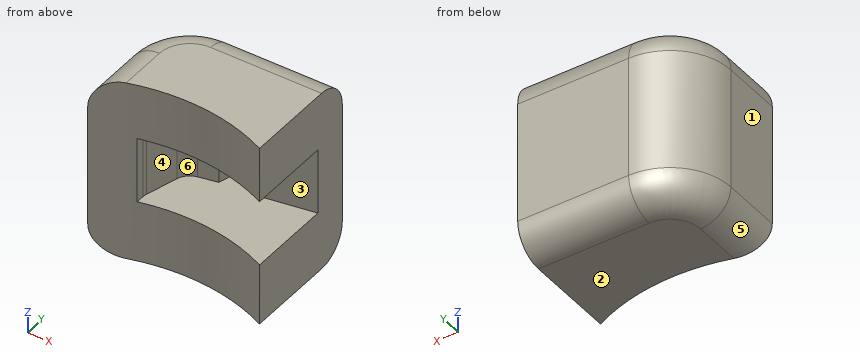
```python
from build123d import *

# Parameters (mm, degrees)
SKETCH1_W                      = 60
SKETCH1_H                      = 60
BOSS_EXTRUDE1_DEPTH            = 40
SKETCH2_R                      = 65
CUT_EXTRUDE1_DEPTH             = 82.241203775
CAVITY1_START                  = -9.816541319
CAVITY1_DEPTH                  = 21.6
SKETCH3_W                      = 21.6
SKETCH3_H                      = 10.847854466
CUT_EXTRUDE2_DEPTH             = 10
SKETCH4_W                      = 60
SKETCH4_H                      = 40
CUT_EXTRUDE3_DEPTH             = 2.5
SKETCH5_W                      = 60
SKETCH5_H                      = 40
CUT_EXTRUDE4_DEPTH             = 1
FILLET1_R                      = 20
FILLET2_R                      = 10
SKETCH6_W                      = 16.032155739
SKETCH6_H                      = 21.6
CUT_EXTRUDE5_DEPTH             = 58.845323025
CUT_EXTRUDE5_DIRECTION_2_REACH = 59.845


# Read off the part's stored shape, not the designer's step: Cavity1
with BuildPart() as part:
    # Sketch1 → Boss-Extrude1 (new body)
    with BuildSketch(Plane(origin=(0, 0, 0), x_dir=(1, 0, 0), z_dir=(0, 1, 0))):
        with Locations((7.418353663, 0)):
            Rectangle(SKETCH1_W, SKETCH1_H)
    extrude(amount=BOSS_EXTRUDE1_DEPTH)

    # Sketch2 → Cut-Extrude1 (cut, through all)
    with BuildSketch(Plane.XY.offset(30)):
        with Locations((8.211917099, -58.463187122)):
            Circle(SKETCH2_R)
    extrude(amount=-CUT_EXTRUDE1_DEPTH, mode=Mode.SUBTRACT)

    # Cavity1 outline → Cavity1 (cut)
    with BuildSketch(Plane.XY.offset(CAVITY1_START)):
        with BuildLine():
            Line((37.418353663, 28.401179965), (19.900272044, 25.583077508))
            Line((19.900272044, 25.583077508), (10.402665556, 28.20897422))
            Line((10.402665556, 28.20897422), (11.046955399, 30.539306317))
            Line((11.046955399, 30.539306317), (8.306376045, 31.297021255))
            Line((8.306376045, 31.297021255), (6.40567059, 24.42235921))
            Line((6.40567059, 24.42235921), (0.254542205, 23.221419402))
            ThreePointArc((0.254542205, 23.221419402), (-2.379423034, 21.883873023), (-3.91543957, 19.360491087))
            Line((-3.91543957, 19.360491087), (-6.809482783, 8.89302545))
            ThreePointArc((-6.809482783, 8.89302545), (-6.970209101, 6.844246899), (-6.353840253, 4.883783703))
            ThreePointArc((-6.353840253, 4.883783703), (14.742582186, 6.207906989), (35.148358053, 0.692777486))
            Line((35.148358053, 0.692777486), (37.418353663, 2.423285883))
            Line((37.418353663, 2.423285883), (37.418353663, 28.401179965))
        make_face()
    extrude(amount=CAVITY1_DEPTH, mode=Mode.SUBTRACT)

    # Sketch3 → Cut-Extrude2 (cut)
    with BuildSketch(Plane(origin=(37.418353663, 0, 0), x_dir=(0, 0, -1), z_dir=(1, 0, 0))):
        with Locations((-0.983458681, 5.423927233)):
            Rectangle(SKETCH3_W, SKETCH3_H)
    extrude(amount=-CUT_EXTRUDE2_DEPTH, mode=Mode.SUBTRACT)

    # Sketch4 → Cut-Extrude3 (cut)
    with BuildSketch(Plane.ZY.offset(22.581646337)):
        with Locations((0, 20)):
            Rectangle(SKETCH4_W, SKETCH4_H)
    extrude(amount=-CUT_EXTRUDE3_DEPTH, mode=Mode.SUBTRACT)

    # Sketch5 → Cut-Extrude4 (cut)
    with BuildSketch(Plane(origin=(37.418353663, 0, 0), x_dir=(0, 0, -1), z_dir=(1, 0, 0))):
        with Locations((0, 20)):
            Rectangle(SKETCH5_W, SKETCH5_H)
    extrude(amount=-CUT_EXTRUDE4_DEPTH, mode=Mode.SUBTRACT)

    # Fillet1
    fillet1_edges = [part.edges().sort_by_distance(p)[0] for p in [
        (-20.081646337, 40, 0),
    ]]
    fillet(fillet1_edges, radius=FILLET1_R)

    # Fillet2
    fillet2_edges = [part.edges().sort_by_distance(p)[0] for p in [
        (-20.081646337, 10.027910314, 30),
        (18.168353663, 40, -30),
        (-20.081646337, 10.027910314, -30),
        (-14.22378196, 34.142135624, -30),
        (18.168353663, 40, 30),
        (-14.22378196, 34.142135624, 30),
    ]]
    fillet(fillet2_edges, radius=FILLET2_R)

    # Sketch6 → Cut-Extrude5 (cut)
    with BuildSketch(Plane(origin=(0, 6.536812878, 0), x_dir=(-1, 0, 0), z_dir=(0, -1, 0))):
        with Locations((-1.011330106, -0.983458681)):
            Rectangle(SKETCH6_W, SKETCH6_H)
    extrude(amount=CUT_EXTRUDE5_DEPTH, mode=Mode.SUBTRACT)

    # Sketch6 → Cut-Extrude5 direction 2 (cut, up to next)
    with BuildSketch(Plane(origin=(0, 6.536812878, 0), x_dir=(-1, 0, 0), z_dir=(0, -1, 0)), mode=Mode.PRIVATE) as cut_extrude5_direction_2_sk1:
        with Locations((-1.011330106, -0.983458681)):
            Rectangle(SKETCH6_W, SKETCH6_H)
    cut_extrude5_direction_2_tool1 = extrude(cut_extrude5_direction_2_sk1.sketch, amount=-CUT_EXTRUDE5_DIRECTION_2_REACH, mode=Mode.PRIVATE) & part.part
    add(cut_extrude5_direction_2_tool1.solids().sort_by_distance((1.01133, 6.536813, 0.983459))[0], mode=Mode.SUBTRACT)


solid = part.part
```
Build history of the part. All positions in model axes, mm. Face numbers are marked on the shaded views. A direction names the side the tool comes from. Round coordinates to 2 decimals unless told otherwise and drop trailing zeros. Write each loop counter-clockwise with the first axis right and the second up, starting at its lowest first coordinate (ties: lowest second). Pieces come first, ordered by that corner, then holes. Notation, with made-up numbers: (15, 69) - (58, 69) arc R8 cw to (58, 75) - close; hole circle Ø8 at (-18.5, -6.75). An arc over 180 degrees is marked (long way). Write each question's results on one line, items separated by ' | '. Start each with the question number.
Item 1: Saw through at B-B (x = 4.5). Write the cut outline in (y, z).
Item 2: Mould opens along Z. For the marked faces 1, 2, 3 and 4 say: pulls with the +Z half, pulls with the -Z half, needs draft (parallel to the pull), parting line crosses it, or undercut.
Item 3: Saw through at A-A (z = -4). Write the cut outline in (x, y).
Item 4: Which spindle directions (+Z, -Z, +X, -X, +Y, -Y) get a long thin tool onto all of the face, cutting with end or side? Do the marked faces 5 and 6. Say none if no direction does.
Item 5: Saw through at C-C (y = 14.5). Write the cut outline in (x, z), and give its area (3 significant figures).
Item 6: Drop flat-ended pins along their axis: P1, Ø1.4, axis at y = 6, z = 2.5, coming from the +X side; P2, Ø1.5, axis at x = 16.5, z = 5, coming from the -Y side; P3, Ø5, axis at x = -6.5, z = 13.5, coming from the +Y side. Give the stop position or say it passes through.
Item 7: Saw through at D-D (z = -16.5). Write the cut outline in (x, y), and give its area (3 significant figures).
Item 8: Wall check: L1, parallel to Z at x = 9.5, y = 9; L2, parallel to X at y = 27.5, z = 19.5; L3, parallel to X at y = 35.5, z = 12. Give the ranges that are in metal, low to high. Write a range as [from, to].
Results are:
1) outline: (6.43, -30) - (30, -30) arc R10 ccw to (40, -20) - (40, 20) arc R10 ccw to (30, 30) - (6.43, 30) - (6.43, 11.78) - (24.05, 11.78) - (24.05, -9.82) - (6.43, -9.82) - close
2) face 1: needs draft | face 2: pulls with the -Z half | face 3: undercut | face 4: undercut
3) outline: (-20.08, 0.06) arc R65 cw to (-7, 4.73) - (-7, 7.45) arc R5.4 cw to (-6.81, 8.89) - (-3.92, 19.36) arc R5.4 cw to (0.25, 23.22) - (6.41, 24.42) - (8.31, 31.3) - (11.05, 30.54) - (10.4, 28.21) - (19.9, 25.58) - (36.42, 28.24) - (36.42, 40) - (-0.08, 40) arc R20 ccw to (-20.08, 20) - close
4) face 5: -Z, -X, +Y, -Y | face 6: +X, -Y
5) outline: (-20.08, -20) arc R10 ccw to (-10.08, -30) - (36.42, -30) - (36.42, -9.82) - (-5.26, -9.82) - (-5.26, 11.78) - (36.42, 11.78) - (36.42, 30) - (-10.08, 30) arc R10 ccw to (-20.08, 20) - close | area: 2,450 mm²
6) P1: stops at x = -7 | P2: stops at y = 26.32 | P3: stops at y = 39.61
7) outline: (-20.08, 0.06) arc R65 cw to (36.42, 0.1) - (36.42, 40) - (-0.08, 40) arc R20 ccw to (-20.08, 20) - close | area: 1,920 mm²
8) L1: z = [-30, -9.82], [11.78, 30] | L2: x = [-18.62, 36.42] | L3: x = [-12.72, 36.42]
